For this review, take the finished solid that the model builds, in its own axes (mm). Face numbers are marked on the shaded views. A direction names the side the tool comes from. Coordinates: 2 decimals unless noted, no trailing zeros. Write each loop counter-clockwise with the first axis right and the second up, starting at its lowest first coordinate (ties: lowest second). Pieces come first, ordered by that corner, then holes.
```python
from build123d import *

# Parameters (mm, degrees)
F0_W      = 59
F0_H      = 59
F1_DEPTH  = 1.5
F3_D      = 3
F3_DEPTH  = 3
F3_TIP    = 0.9012909285
F2_W      = 27
F2_H      = 45
F4_DEPTH  = 11
F2_W_2    = 7
F2_H_2    = 22.5
F5_DEPTH  = 25
F2_W_3    = 15
F2_H_3    = 5.6414641738
F6_DEPTH  = 16
F2_W_4    = 16.4975724295
F2_H_4    = 16.1418512762
F7_DEPTH  = 16
F2_W_5    = 15.5616942793
F2_H_5    = 8
F8_DEPTH  = 25
F2_W_6    = 5
F9_DEPTH  = 6
F2_R      = 3.1285701803
F10_DEPTH = 12
F11_W     = 5
F11_H     = 6
F12_DEPTH = 2
F14_D     = 3
F14_DEPTH = 6
F14_TIP   = 0.9012909285
F2_W_7    = 8
F15_DEPTH = 4
F16_W     = 8
F16_H     = 4
F17_DEPTH = 2
F2_R_2    = 2.591599319
F18_DEPTH = 10


with BuildPart() as f1:
    # F0 (on Top) → F1 (new body)
    with BuildSketch(Plane.XY):
        Rectangle(F0_W, F0_H)
    extrude(amount=F1_DEPTH)

    # F3
    with Locations(Plane.XY.offset(1.5)):
        with Locations((26.8, -26.9), (-27.2, -26.9), (-27.2, 27.1), (26.8, 27.1)):
            Hole(F3_D / 2, depth=F3_DEPTH)
            with Locations((0, 0, -(F3_DEPTH + F3_TIP / 2))):  # 118° drill point
                Cone(0, F3_D / 2, F3_TIP, mode=Mode.SUBTRACT)

    # F2 (on face) → F4 (join)
    with BuildSketch(Plane.XY.offset(1.5)):
        with Locations((5, 7)):
            Rectangle(F2_W, F2_H)
    extrude(amount=F4_DEPTH)

    # F2 (on face) → F5 (join)
    with BuildSketch(Plane.XY.offset(1.5)):
        with Locations((23, -5.75)):
            Rectangle(F2_W_2, F2_H_2)
    extrude(amount=F5_DEPTH)

    # F2 (on face) → F6 (join)
    with BuildSketch(Plane.XY.offset(1.5)):
        with Locations((-17, 21.6792679131)):
            Rectangle(F2_W_3, F2_H_3)
    extrude(amount=F6_DEPTH)

    # F2 (on face) → F7 (join)
    with BuildSketch(Plane.XY.offset(1.5)):
        with Locations((-17.9585402422, 9.7876101881)):
            Rectangle(F2_W_4, F2_H_4)
    extrude(amount=F7_DEPTH)

    # F2 (on face) → F8 (join)
    with BuildSketch(Plane.XY.offset(1.5)):
        with Locations((-17.0449977741, -3.5)):
            Rectangle(F2_W_5, F2_H_5)
    extrude(amount=F8_DEPTH)

    # F2 (on face) → F9 (join)
    with BuildSketch(Plane.XY.offset(1.5)):
        with Locations((-16.5, -25.5)):
            Rectangle(F2_W_6, F2_H_5)
        with Locations((-17.0449977741, -3.5)):
            Rectangle(F2_W_5, F2_H_5)
    extrude(amount=F9_DEPTH)

    # F2 (on face) → F10 (join)
    with BuildSketch(Plane.XY.offset(1.5)):
        with Locations((24.5, -20.9337305278)):
            Circle(F2_R)
    extrude(amount=F10_DEPTH)

    # F11 (on face) → F12 (join)
    with BuildSketch(Plane.XZ.offset(29.5)):
        with Locations((-16.5, 4.5)):
            Rectangle(F11_W, F11_H)
    extrude(amount=F12_DEPTH)

    # F14
    with Locations(Plane.XZ.offset(31.5)):
        with Locations((-16.4128988981, 4.5567261986)):
            Hole(F14_D / 2, depth=F14_DEPTH)
            with Locations((0, 0, -(F14_DEPTH + F14_TIP / 2))):  # 118° drill point
                Cone(0, F14_D / 2, F14_TIP, mode=Mode.SUBTRACT)

    # F2 (on face) → F15 (join)
    with BuildSketch(Plane.XY.offset(1.5)):
        with Locations((11.5, -25.5)):
            Rectangle(F2_W_7, F2_H_5)
    extrude(amount=F15_DEPTH)

    # F16 (on face) → F17 (join)
    with BuildSketch(Plane.XZ.offset(29.5)):
        with Locations((11.5, 3.5)):
            Rectangle(F16_W, F16_H)
    extrude(amount=F17_DEPTH)

    # F2 (on face) → F18 (join)
    with BuildSketch(Plane.XY.offset(1.5)):
        with Locations((3.5, -18.7545120716)):
            Circle(F2_R_2)
    extrude(amount=F18_DEPTH)


solid = f1.part
```
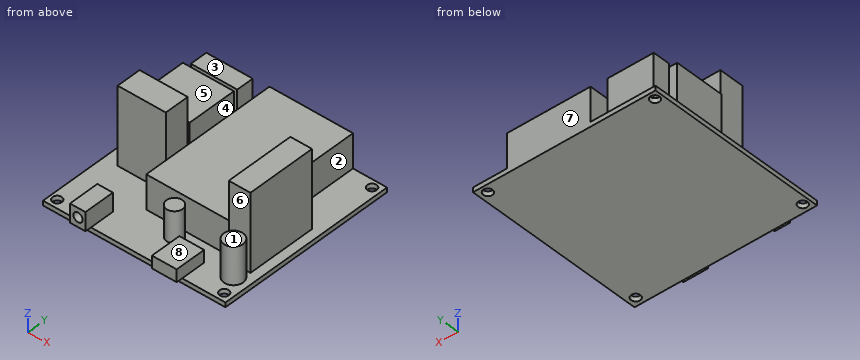
Q1. Add section D-D (y = -26.9). State the section outline as (x, z) points, then the cut area to 3 significant figures.
Ans:
outline: (-29.5, 0) - (-28.7, 0) - (-28.7, 1.5) - (-29.5, 1.5) - close; (-25.7, 0) - (25.3, 0) - (25.3, 1.5) - (15.5, 1.5) - (15.5, 5.5) - (7.5, 5.5) - (7.5, 1.5) - (-14, 1.5) - (-14, 7.5) - (-19, 7.5) - (-19, 1.5) - (-25.7, 1.5) - close; (28.3, 0) - (29.5, 0) - (29.5, 1.5) - (28.3, 1.5) - close; hole circle Ø3 at (-16.41, 4.56)
area: 134 mm2
Q2. Add section C-C (z = 19.5). State the section outline as (x, y) points, then the cut area to 3 significant figures.
Ans:
outline: (-24.83, -7.5) - (-9.26, -7.5) - (-9.26, 0.5) - (-24.83, 0.5) - close; (19.5, -17) - (26.5, -17) - (26.5, 5.5) - (19.5, 5.5) - close
area: 282 mm2
Q3. Add section B-B (x = 24.5). State the section outline as (y, z) points.
Ans:
outline: (-29.5, 0) - (29.5, 0) - (29.5, 1.5) - (5.5, 1.5) - (5.5, 26.5) - (-17, 26.5) - (-17, 1.5) - (-17.81, 1.5) - (-17.81, 13.5) - (-24.06, 13.5) - (-24.06, 1.5) - (-29.5, 1.5) - close
Q4. Add section A-A (y = 27.1). State the section outline as (x, z) points.
Ans:
outline: (-29.5, 0) - (-28.7, 0) - (-28.7, 1.5) - (-29.5, 1.5) - close; (-25.7, 0) - (25.3, 0) - (25.3, 1.5) - (18.5, 1.5) - (18.5, 12.5) - (-8.5, 12.5) - (-8.5, 1.5) - (-25.7, 1.5) - close; (28.3, 0) - (29.5, 0) - (29.5, 1.5) - (28.3, 1.5) - close
Q5. Tool access review of the marked faces 1, 2, 3, 4 and 5: name each direction out of +Z, -Z, +X, -X, +Y, -Y from which nothing blocks a thin tool from reaching the whole face with its end or side.
Ans:
face 1: +Z, +X, -X, -Y
face 2: +Z, +Y, -Y
face 3: +Z, +X, -X, +Y
face 4: +Z
face 5: +Z, -X, +Y
Q6. For probe 1 along Y at (x, z) = (-27.2, 0.75); probe 2 along Y at (x, z) = (-21, 13.25); probe 3 along X at (y, z) = (20.5, 10.5), list the stretches that pass through material, from the lowest coordinate up.
Ans:
probe 1: y = -29.5 to -28.4, -25.4 to 25.6, 28.6 to 29.5
probe 2: y = -7.5 to 0.5, 1.72 to 17.86, 18.86 to 24.5
probe 3: x = -24.5 to -9.5, -8.5 to 18.5
Q7. Clearance check with flat-ended pins moving along their axes: pin 1 Ø2 at (y, z) = (-25, 4) entering from -X; pin 2 Ø6.5 at (x, y) = (12, -25.5) entering from +Z; pin 3 Ø8 at (x, z) = (3, 11.5) entering from -Y; pin 4 Ø6 at (x, y) = (-1.5, -17) entering from -Z. State where each tip first meets the part, or that it passes through.
Ans:
pin 1: stops at x = -19
pin 2: stops at z = 5.5
pin 3: stops at y = -21.35
pin 4: stops at z = 0
Q8. Draft analysis for pull direction Y (two halves, no side actions). For the marked faces 6, 7 and 8, state which applies: +Y half, -Y half, draft (parallel to the pull), parting line (faces both ways), or undercut.
Ans:
face 6: undercut
face 7: +Y half
face 8: draft
